Could you check a few things on this model? Use its own coordinates, in mm. Coordinates: 2 decimals unless noted, no trailing zeros. Order: outer loops, then holes, each group sorted by start corner. A loop starts at its lowest first (then second) coordinate and runs counter-clockwise, first axis right, second up. Notation, with made-up numbers: M 50.5,78 L 91.5,78 A20 ccw 91.5,112 Z; hole C 2.25,59 d1. An arc over 180 degrees is marked long. Write item = value, one per line. Start each with the question number.
Autodesk Inventor part; units mm, degrees
ref_plane "YZ Plane" through (0, 0, 0) normal (1, 0, 0) x (0, 1, 0)
ref_plane "XZ Plane" through (0, 0, 0) normal (0, 1, 0) x (-1, 0, 0)
ref_plane "XY Plane" through (0, 0, 0) normal (0, 0, 1) x (1, 0, 0)
sketch "Sketch1" plane through (0, 0, 0) normal (0, 0, 1) x (1, 0, 0)
  line L0 (0, 0) -> (780, 0)
  line L1 (780, 0) -> (780, 21)
  line L2 (780, 21) -> (0, 21)
  line L3 (0, 21) -> (0, 0)
  dimension "d0" = 780
  dimension "d1" = 21
extrude "Extrusion1" add sketch "Sketch1" along normal blind 80
sketch "Sketch2" plane through (0, 21, 0) normal (0, 1, 0) x (1, 0, 0)
  line L0 (780, 0) -> (780, -80)
  line L1 (780, 0) -> (680, 0)
  line L2 (680, 0) -> (680, -25)
  line L3 (680, -25) -> (780, -25)
  line L4 (780, -25) -> (780, 0)
  point P0 (0, 0)
  dimension "d4" = 100
  dimension "d5" = 25
extrude "Extrusion2" cut sketch "Sketch2" against normal through all
properties part number "MPX-rib2" material "Wood (Cherry)"
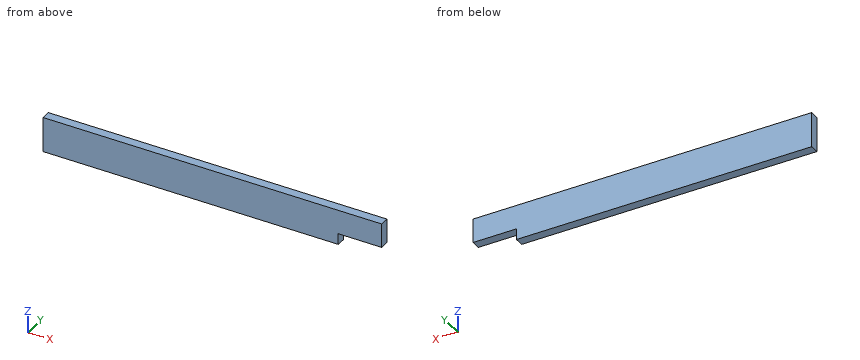
(1) Imagine slicing it at A-A on y = 6. List the corners of the cut face in (x, z) for me.
(2) Imagine slicing it at B-B on x = 691. List the corners of the cut face in (y, z) for me.
(3) Please list where these lines run through material, in increasing order: probe 1 along Z at (x, y) = (687.5, 19.5); probe 2 along X at (y, z) = (3, 13). Write a range as from..to.
(4) Will these pins go through, and if not, where does the flat tip stop? P1, Ø6, axis at x = 458.5, y = 6.5, coming from the -Z side; P2, Ø6.5, axis at x = 728.5, y = 9, coming from the -Z side.
Response:
q1.outline = M 0,0 L 680,0 L 680,25 L 780,25 L 780,80 L 0,80 Z
q2.outline = M 0,25 L 21,25 L 21,80 L 0,80 Z
q3.probe_1 = 25..80
q3.probe_2 = 0..680
q4.P1 = 0
q4.P2 = 25
